from build123d import *

# Parameters (mm, degrees)
F2_R     = 7.375
F3_DEPTH = 3
F4_SIZE  = 0.5


with BuildPart() as f1:
    # F0 (on Front) → F1 (revolve)
    with BuildSketch(Plane.XZ):
        Polygon((7.375, 3), (3.3, 3), (3.3, 0), (6, 0), (7.5, -4), (10, -4), align=None)
    revolve(axis=Axis((0, 0, -0.17444), (0, 0, 1)))

    # F2 (on face) → F3 (join)
    with BuildSketch(Plane.XY.offset(3)):
        Circle(F2_R)
        with BuildLine():
            ThreePointArc((-0.5, 5.715768), (0, 5.849742), (0.5, 5.715768))
            Line((0.5, 5.715768), (4.7, 3.290897))
            ThreePointArc((4.7, 3.290897), (5.066025, 2.924871), (5.2, 2.424871))
            Line((5.2, 2.424871), (5.2, -2.424871))
            ThreePointArc((5.2, -2.424871), (5.066025, -2.924871), (4.7, -3.290897))
            Line((4.7, -3.290897), (0.5, -5.715768))
            ThreePointArc((0.5, -5.715768), (0, -5.849742), (-0.5, -5.715768))
            Line((-0.5, -5.715768), (-4.7, -3.290897))
            ThreePointArc((-4.7, -3.290897), (-5.066025, -2.924871), (-5.2, -2.424871))
            Line((-5.2, -2.424871), (-5.2, 2.424871))
            ThreePointArc((-5.2, 2.424871), (-5.066025, 2.924871), (-4.7, 3.290897))
            Line((-4.7, 3.290897), (-0.5, 5.715768))
        make_face(mode=Mode.SUBTRACT)
    extrude(amount=F3_DEPTH)

    # F4
    f4_edges = [f1.edges().sort_by_distance(p)[0] for p in [
        (-5.2, 0, 6),
    ]]
    chamfer(f4_edges, length=F4_SIZE)


solid = f1.part
The model under review builds one solid part; all positions refer to its coordinate system, in mm. A direction names the side the tool comes from. Round coordinates to 2 decimals unless told otherwise and drop trailing zeros. Order: outer loops, then holes, each group sorted by start corner. A loop starts at its lowest first (then second) coordinate and runs counter-clockwise, first axis right, second up. Notation, with made-up numbers: (45.5, 89) -> (84.5, 89) arc R29 ccw to (84.5, 123) -> close; hole circle Ø1 at (5.25, 88.5). An arc over 180 degrees is marked (long way). Return JSON: item names as keys, results as strings.
1. Take a section at B-B (x = 0). Write out the cut boundary in (y, z) (3 decimals).
Answer block:
{"outline": "(-10, -4) -> (-7.5, -4) -> (-6, 0) -> (-3.3, 0) -> (-3.3, 3) -> (-5.85, 3) -> (-5.85, 5.5) -> (-6.35, 6) -> (-7.375, 6) -> (-7.375, 3) -> close; (3.3, 0) -> (6, 0) -> (7.5, -4) -> (10, -4) -> (7.375, 3) -> (7.375, 6) -> (6.35, 6) -> (5.85, 5.5) -> (5.85, 3) -> (3.3, 3) -> close"}
2. For faces 4 (the face through (-5.2, 0, 4)), 5 (the face through (5.812, 1.83, -0.25)), list the 3-axis set-ups (+Z, -Z, +X, -X, +Y, -Y) from which the entire face can be reached by the end or side of a thin tool; tool diameter is ignored.
Answer block:
{"face 4": "+Z", "face 5": "-Z"}
3. For L1, parallel to X at y = 0.75, z = 3.25; L2, parallel to Y at x = 0, z = 1.25; L3, parallel to Z at x = 2.75, y = -3.75, list the stretches that pass through material, from the lowest coordinate up. Write a range as [from, to].
Answer block:
{"L1": "x = [-7.34, -5.2], [5.2, 7.34]", "L2": "y = [-8.03, -3.3], [3.3, 8.03]", "L3": "z = [0, 3]"}
4. The part is to be moulded in two halves that separate along X. For faces 1 (the face through (6.93, -2.87, 2.66)), 2 (the face through (-2.753, 4.7, 5.746)), 3 (the face through (-4, 7, -4)), say which applies: +X half, -X half, draft (parallel to the pull), parting line (faces both ways), or undercut.
Answer block:
{"face 1": "parting line", "face 2": "undercut", "face 3": "draft"}
5. Insertion check: P1, Ø0.8, axis at y = -0.5, z = 4, coming from the -X side; P2, Ø6, axis at x = -2, z = 0, coming from the +Y side; P3, Ø4, axis at x = 0.5, y = 2, coming from the -Z side; P4, Ø1, axis at x = -2.5, y = -0.5, coming from the -Z side. Each pin has a flat end and moves straight along its axis. Give the tip position at first contact, or say it passes through.
Answer block:
{"P1": "stops at x = -7.37", "P2": "stops at y = 9.51", "P3": "stops at z = 0", "P4": "passes through"}
6. Take a section at C-C (y = 0). Write out the cut boundary in (x, z) (3 decimals), then the cut area to 3 significant figures.
Answer block:
{"outline": "(-10, -4) -> (-7.5, -4) -> (-6, 0) -> (-3.3, 0) -> (-3.3, 3) -> (-5.2, 3) -> (-5.2, 5.5) -> (-5.7, 6) -> (-7.375, 6) -> (-7.375, 3) -> close; (3.3, 0) -> (6, 0) -> (7.5, -4) -> (10, -4) -> (7.375, 3) -> (7.375, 6) -> (5.7, 6) -> (5.2, 5.5) -> (5.2, 3) -> (3.3, 3) -> close", "area": "60.6 mm²"}
7. Take a section at D-D (z = -0.25). Write out the cut boundary in (x, y), then the cut area to 3 significant figures.
Answer block:
{"outline": "circle Ø17.19 at (0, 0); hole circle Ø12.19 at (0, 0)", "area": "115 mm²"}
8. Take a section at A-A (z = 3.75). Write out the cut boundary in (x, y) (3 decimals).
Answer block:
{"outline": "circle Ø14.75 at (0, 0); hole (-5.2, -2.425) arc R1 ccw to (-4.7, -3.291) -> (-0.5, -5.716) arc R1 ccw to (0.5, -5.716) -> (4.7, -3.291) arc R1 ccw to (5.2, -2.425) -> (5.2, 2.425) arc R1 ccw to (4.7, 3.291) -> (0.5, 5.716) arc R1 ccw to (-0.5, 5.716) -> (-4.7, 3.291) arc R1 ccw to (-5.2, 2.425) -> close"}
